from build123d import *

# Parameters (mm, degrees)
F1_DEPTH = 34


with BuildPart() as f1:
    # F0 (on Top) → F1 (new body)
    with BuildSketch(Plane.XY):
        with BuildLine():
            ThreePointArc((-72, 7), (-69.949747, 2.050253), (-65, 0))
            ThreePointArc((-65, 0), (-60.050253, 2.050253), (-58, 7))
            ThreePointArc((-58, 7), (-60.050253, 11.949747), (-65, 14))
            ThreePointArc((-65, 14), (-69.949747, 11.949747), (-72, 7))
        make_face()
        with BuildLine():
            Line((-65, 0), (-7, 0))
            ThreePointArc((-7, 0), (-14, 7), (-7, 14))
            Line((-7, 14), (-65, 14))
            ThreePointArc((-65, 14), (-60.050253, 11.949747), (-58, 7))
            ThreePointArc((-58, 7), (-60.050253, 2.050253), (-65, 0))
        make_face()
        with BuildLine():
            ThreePointArc((-7, 14), (-14, 7), (-7, 0))
            ThreePointArc((-7, 0), (-2.050253, 2.050253), (0, 7))
            ThreePointArc((0, 7), (-2.050253, 11.949747), (-7, 14))
        make_face()
    extrude(amount=F1_DEPTH)


solid = f1.part
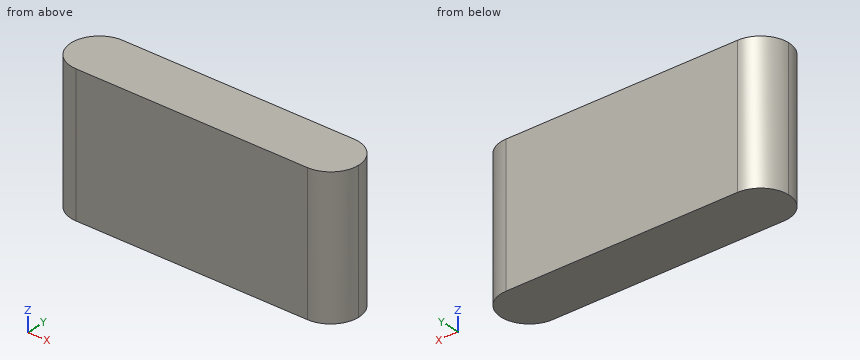
Verification items for the finished model (mm, model axes). Coordinates: 2 decimals unless noted, no trailing zeros. Order: outer loops, then holes, each group sorted by start corner. A loop starts at its lowest first (then second) coordinate and runs counter-clockwise, first axis right, second up.
1. Sectioned sample at B-B, the plane y = 1.5. Record the cut outline in (x, z).
Results found:
outline: (-69.33, 0) - (-2.67, 0) - (-2.67, 34) - (-69.33, 34) - close
2. Sectioned sample at A-A, the plane z = 21. Record the cut outline in (x, y).
Results found:
outline: (-72, 7) arc R7 ccw to (-65, 0) - (-7, 0) arc R7 ccw to (0, 7) arc R7 ccw to (-7, 14) - (-65, 14) arc R7 ccw to start
3. Scan lines: line 1 (X direction, y = 9, z = 28); line 2 (X direction, y = 12.75, z = 15); line 3 (Y direction, x = -68, z = 24.5). Record each from-to range of solid material in increasing order.
Results found:
line 1: x = -71.71 to -0.29
line 2: x = -68.99 to -3.01
line 3: y = 0.68 to 13.32
4. Go/stop test with flat-tipped pins: pin 1 Ø1.5 at (y, z) = (6.5, 9.5) entering from +X; pin 2 Ø4 at (y, z) = (2, 5) entering from +X; pin 3 Ø2 at (y, z) = (2, 17) entering from -X. Record where each tip stops, or that it passes through.
Results found:
pin 1: stops at x = 0
pin 2: stops at x = -0.68
pin 3: stops at x = -70.74
5. Sectioned sample at C-C, the plane x = -5.5. Record the cut outline in (y, z), and give its area (3 significant figures).
Results found:
outline: (0.16, 0) - (13.84, 0) - (13.84, 34) - (0.16, 34) - close
area: 465 mm2
